from build123d import *

# Parameters (mm, degrees)
F2_R = 0.5


with BuildPart() as f1:
    # F0 (on Front) → F1 (revolve)
    with BuildSketch(Plane.XZ):
        with BuildLine():
            Line((-4.9, 7.563289), (-4.033975, 8.063289))
            ThreePointArc((-4.033975, 8.063289), (-3.899296, 8.197967), (-3.85, 8.381942))
            Line((-3.85, 8.381942), (-3.85, 10.523096))
            Line((-3.85, 10.523096), (-5.35, 10.523096))
            Line((-5.35, 10.523096), (-5.35, 7.823096))
            ThreePointArc((-5.35, 7.823096), (-5.2, 7.563289), (-4.9, 7.563289))
        make_face()
    revolve(axis=Axis((0, 0, -0.587365), (0, 0, -1)))

    # F2
    f2_edges = [f1.edges().sort_by_distance(p)[0] for p in [
        (3.85, 0, 10.523096),
        (5.35, 0, 10.523096),
    ]]
    fillet(f2_edges, radius=F2_R)


solid = f1.part
The listing builds one solid part. Answer for the finished solid, in the listing's coordinates (mm). Coordinates: 2 decimals unless noted, no trailing zeros. Write each loop counter-clockwise with the first axis right and the second up, starting at its lowest first coordinate (ties: lowest second). Pieces come first, ordered by that corner, then holes. Notation, with made-up numbers: M 87,79.5 L 104,79.5 A10 ccw 104,96.5 Z; hole C 74,89.25 d7. An arc over 180 degrees is marked long. Put each result on its own line as item: value. Start each with the question number.
1. Flat-ended cylindrical pins translate along their axes: P1, Ø4, axis at x = 1, y = -2, coming from the -Z side; P2, Ø5, axis at x = -1, y = 0.5, coming from the -Z side; P3, Ø1.5, axis at x = -1, z = 8.5, coming from the -Y side; P4, Ø3, axis at x = 4, y = 1.5, coming from the +Z side. Find the tip coordinate at first contact, or state that the pin passes through.
2. A cutting plane is placed at A-A on x = 0. Write down the section's boundary in (y, z).
3. A cutting plane is placed at C-C on z = 9.8. Write down the section's boundary in (x, y), then the cut area to 3 significant figures.
4. For a pull along Y with two mould halves and no side action, classify faces 1 (the cylindrical face through (0.83, -3.76, 9.21)), 2 (the cylindrical face through (1.16, -5.223, 8.908)) as pulls with the +Y half, pulls with the -Y half, needs draft (parallel to the pull), parting line crosses it, or undercut.
5. Consider line 1 (Y direction, x = 0, z = 10.05); line 2 (X direction, y = 2.25, z = 8.35). Determine where each line is inside the solid, lowest interval first. Write a range as from..to.
Resolved:
1. P1: stops at z = 7.95
1. P2: passes through
1. P3: stops at y = -5.34
1. P4: stops at z = 10.52
2. outline: M -5.35,7.82 A0.3 ccw -4.9,7.56 L -4.03,8.06 A0.37 ccw -3.85,8.38 L -3.85,10.02 A0.5 ccw -4.35,10.52 L -4.85,10.52 A0.5 ccw -5.35,10.02 Z; M 3.85,8.38 A0.37 ccw 4.03,8.06 L 4.9,7.56 A0.3 ccw 5.35,7.82 L 5.35,10.02 A0.5 ccw 4.85,10.52 L 4.35,10.52 A0.5 ccw 3.85,10.02 Z
3. outline: C 0,0 d10.7; hole C 0,0 d7.7
3. area: 43.4 mm2
4. face 1: undercut
4. face 2: parting line crosses it
5. line 1: y = -5.35..-3.85, 3.85..5.35
5. line 2: x = -4.85..-3.13, 3.13..4.85
